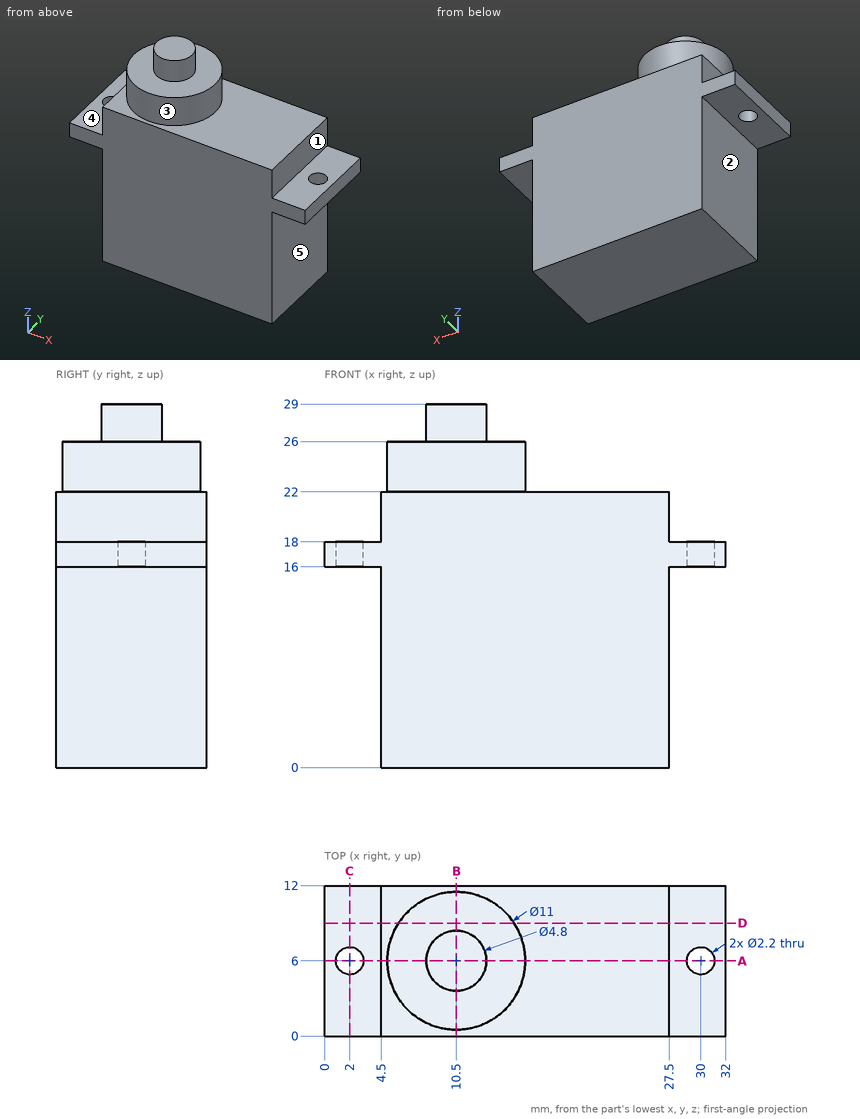
Study the drawing (mm; zero at the part's minimum x, y, z) and answer. A direction names the side the tool comes from. Round coordinates to 2 decimals unless told otherwise and drop trailing zeros. Order: outer loops, then holes, each group sorted by start corner. A loop starts at its lowest first (then second) coordinate and runs counter-clockwise, first axis right, second up. Notation, with made-up numbers: (-29.5, 33) -> (-4.5, 33) arc R26 ccw to (-4.5, 59) -> close; hole circle Ø4 at (-8.5, -25). An arc over 180 degrees is marked (long way). Answer as CSV lines item,"result". Start each with the question number.
(1) Flat-ended cylindrical pins translate along their axes: pin 1 Ø2 at (y, z) = (5, 25) entering from +X; pin 2 Ø3 at (x, y) = (8, 11) entering from +Z; pin 3 Ø3 at (y, z) = (5, 6) entering from +X. Find the tip coordinate at first contact, or state that the pin passes through.
(2) The part is cut by section C-C (x = 2). Determine the outline of the cut face in (y, z).
(3) The part is cut by section D-D (y = 9). Determine the outline of the cut face in (x, z).
(4) A tool of negligible diameter and unlimited length cuts with its end or side. For the marked faces 1, 2, 3, 4 and 5, from which of +Z, -Z, +X, -X, +Y, -Y can it reach the whole face along a straight path? Write none if from no direction.
(5) Find the intervals of material crossed by probe 1 along X at (y, z) = (6, 17.55); probe 2 along Y at (x, z) = (2, 16.8); probe 3 along Z at (x, y) = (28.5, 4.5), in increasing order. Write a range as from..to.
(6) The part is cut by section A-A (y = 6). Determine the outline of the cut face in (x, z), then the cut area to 3 significant figures.
(7) The part is cut by section B-B (x = 10.5). Determine the outline of the cut face in (y, z), then the cut area to 3 significant figures.
Evaluation:
1,pin 1,"x = 16"
1,pin 2,"z = 26"
1,pin 3,"x = 27.5"
2,outline,"(0, 16) -> (4.9, 16) -> (4.9, 18) -> (0, 18) -> close; (7.1, 16) -> (12, 16) -> (12, 18) -> (7.1, 18) -> close"
3,outline,"(0, 16) -> (4.5, 16) -> (4.5, 0) -> (27.5, 0) -> (27.5, 16) -> (32, 16) -> (32, 18) -> (27.5, 18) -> (27.5, 22) -> (15.11, 22) -> (15.11, 26) -> (5.89, 26) -> (5.89, 22) -> (4.5, 22) -> (4.5, 18) -> (0, 18) -> close"
4,face 1,"+Z, +X, +Y, -Y"
4,face 2,"-Z, -X, +Y, -Y"
4,face 3,"+Z"
4,face 4,"+Z, -X, +Y, -Y"
4,face 5,"-Z, +X, +Y, -Y"
5,probe 1,"0..0.9, 3.1..28.9, 31.1..32"
5,probe 2,"0..4.9, 7.1..12"
5,probe 3,"16..18"
6,outline,"(0, 16) -> (0.9, 16) -> (0.9, 18) -> (0, 18) -> close; (3.1, 16) -> (4.5, 16) -> (4.5, 0) -> (27.5, 0) -> (27.5, 16) -> (28.9, 16) -> (28.9, 18) -> (27.5, 18) -> (27.5, 22) -> (16, 22) -> (16, 26) -> (12.9, 26) -> (12.9, 29) -> (8.1, 29) -> (8.1, 26) -> (5, 26) -> (5, 22) -> (4.5, 22) -> (4.5, 18) -> (3.1, 18) -> close; (31.1, 16) -> (32, 16) -> (32, 18) -> (31.1, 18) -> close"
6,area,"574 mm²"
7,outline,"(0, 0) -> (12, 0) -> (12, 22) -> (11.5, 22) -> (11.5, 26) -> (8.4, 26) -> (8.4, 29) -> (3.6, 29) -> (3.6, 26) -> (0.5, 26) -> (0.5, 22) -> (0, 22) -> close"
7,area,"322 mm²"
